Geometry check sheet. Reference: the model listing, model coordinates, mm. A direction names the side the tool comes from. Give positions to 0.01 mm unless a question says otherwise; leave off trailing zeros. Write each loop counter-clockwise with the first axis right and the second up, starting at its lowest first coordinate (ties: lowest second). Pieces come first, ordered by that corner, then holes. Notation, with made-up numbers: M 73,42.5 L 107,42.5 A13 cw 107,58.5 Z; hole C -32,-4 d4. An arc over 180 degrees is marked long. One line per item, written item: value. Start each with the question number.
1. Tool access check on faces 1 (the face through (-251, 8, -52)), 2 (the face through (-252.833, 6.028, -52.359)), 3 (the face through (-274.94, 5.92, -3.04)). Record the directions out of +Z, -Z, +X, -X, +Y, -Y that give a thin tool (end or side, any length) a straight path to the whole face; none if there is none.
2. Release check for a two-part mould opening along Z. For faces 4 (the face through (-287.287, 6.028, -61.223)), 5 (the face through (-288, 8, -59)), 6 (the face through (-275, 6, 0)), 7 (the face through (-259.13, 5.92, -12.88)) record: pulls with the +Z half, pulls with the -Z half, needs draft (parallel to the pull), parting line crosses it, or undercut.
3. Cross-section at C-C on z = -11.5. Record the cut outline in (x, y).
4. Gauge pin test, flat ends, axial feed: pin 1 (4 mm diameter, centred on x = -250.5, z = -53, fed in from -Y); pin 2 (4 mm diameter, centred on y = 7, z = -25, fed in from -X); pin 3 (4 mm diameter, centred on x = -251.5, z = -52.5, fed in from +Y). Record the tip position at first contact, or that the pin passes through.
5. Scan lines: line 1 (Z direction, x = -275, y = 9.75); line 2 (Z direction, x = -273, y = 1.75); line 3 (X direction, y = 4.5, z = -35.5). Record each from-to range of solid material in increasing order.
6. Cross-section at B-B on x = -262.5. Record the cut outline in (y, z).
7. Cross-section at A-A on y = 6.25. Count the separate pieces of the cut face and the enclosed holes in it, then the cut area to 3 significant figures.
8. Cross-section at D-D on x = -271. Record the cut outline in (y, z), then the cut area to 3 significant figures.
from build123d import *

# Parameters (mm, degrees)
BOSS_EXTRUDE1_DEPTH = 12
BOSS_EXTRUDE2_DEPTH = 3


with BuildPart() as part:
    # Sketch1 → Boss-Extrude1 (new body)
    with BuildSketch(Plane(origin=(0, 0, 0), x_dir=(1, 0, 0), z_dir=(0, 1, 0))):
        with BuildLine():
            Line((-289.517864278, 57.588683782), (-250.286431131, 49.785066539))
            ThreePointArc((-250.286431131, 49.785066539), (-253.961023409, 25.012977594), (-255.189832201, 0))
            Line((-255.189832201, 0), (-295.127762341, 0))
            Line((-295.127762341, 0), (-295.127762341, 6.054265565))
            ThreePointArc((-295.127762341, 6.054265565), (-293.456259512, 31.944858577), (-289.517864278, 57.588683782))
        make_face()
        Polygon((-255.364905165, 48.501157726), (-258.362561508, 27.716209892), (-289.038525769, 32.186692712), (-286.040869426, 52.971640546), align=None, mode=Mode.SUBTRACT)
        Polygon((-258.596218965, 23.222280187), (-259.674858729, 2.25), (-290.633540871, 3.85), (-289.554901108, 24.822280187), align=None, mode=Mode.SUBTRACT)
    extrude(amount=BOSS_EXTRUDE1_DEPTH)

    # Sketch4 → Boss-Extrude2 (add)
    with BuildSketch(Plane(origin=(-250.286431131, 0, -49.785066539), x_dir=(0.19509032201612864, 0, -0.9807852804032304), z_dir=(0.9807852804032303, 0, 0.1950903220161286))):
        Polygon((-0.699680901, 12), (0, 12), (0, 8), (4, 8), (4, 4), (0, 4), (0, 0), (-0.699680901, 0), align=None)
    boss_extrude2 = extrude(amount=-BOSS_EXTRUDE2_DEPTH)

    # Mirror3: Boss-Extrude2 across plane
    add(boss_extrude2.mirror(Plane(origin=(-269.902136739, 0, -53.68687298), x_dir=(-0.19509032201612864, 0, 0.9807852804032303), z_dir=(0.9807852804032304, 0, 0.19509032201612864))))


solid = part.part
Report:
1. face 1: -Z, +X, +Y
1. face 2: -Z, +Y, -Y
1. face 3: +Y, -Y
2. face 4: pulls with the -Z half
2. face 5: needs draft
2. face 6: pulls with the +Z half
2. face 7: undercut
3. outline: M -294.97,0 L -290.24,0 L -290.24,12 L -294.97,12 Z; M -259.2,0 L -254.93,0 L -254.93,12 L -259.2,12 Z
4. pin 1: stops at y = 4
4. pin 2: stops at x = -294.29
4. pin 3: stops at y = 8
5. line 1: z = -54.7 to -51.36, -30.14 to -24.07, -3.04 to 0
5. line 2: z = -54.3 to -51.07, -29.85 to -23.97, -2.94 to 0
5. line 3: x = -293.05 to -288.56, -257.24 to -252.71
6. outline: M 0,-52.21 L 12,-52.21 L 12,-49.54 L 0,-49.54 Z; M 0,-28.32 L 12,-28.32 L 12,-23.42 L 0,-23.42 Z; M 0,-2.4 L 12,-2.4 L 12,0 L 0,0 Z
7. separate pieces: 1
7. enclosed holes: 2
7. area: 883 mm^2
8. outline: M 0,-53.91 L 12,-53.91 L 12,-50.78 L 0,-50.78 Z; M 0,-29.56 L 12,-29.56 L 12,-23.86 L 0,-23.86 Z; M 0,-2.84 L 12,-2.84 L 12,0 L 0,0 Z
8. area: 140 mm^2
